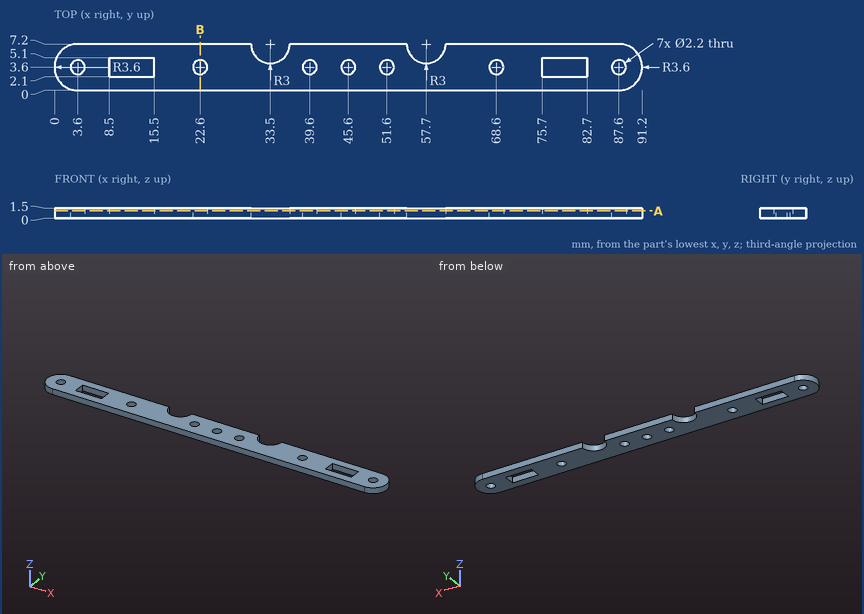
The figure shows three views and two pictorial views of one solid part (mm, origin at its lowest corner). Answer the questions. Coordinates: 2 decimals unless noted, no trailing zeros. Order: outer loops, then holes, each group sorted by start corner. A loop starts at its lowest first (then second) coordinate and runs counter-clockwise, first axis right, second up. Notation, with made-up numbers: (56, 66) - (76, 66) arc R19 cw to (76, 83) - close; hole circle Ø1 at (49.5, -5.75). An arc over 180 degrees is marked (long way). Answer as a JSON object with one key per item and string values.
1. Find section A-A on z = 1.1. Count the separate pieces of the cut face and the enclosed holes in it, plus the area to 3 significant figures.
Output values:
{"separate pieces": "1", "enclosed holes": "9", "area": "549 mm²"}
2. Consider line 1 (Y direction, x = 45.6, z = 0.45); line 2 (X direction, y = 5, z = 1.2); line 3 (Y direction, x = 9, z = 0.3). Determine where each line is inside the solid, lowest interval first.
Output values:
{"line 1": "y = 0 to 2.5, 4.7 to 7.2", "line 2": "x = 0.28 to 8.5, 15.5 to 31.46, 35.54 to 55.66, 59.74 to 75.7, 82.7 to 90.92", "line 3": "y = 0 to 2.1, 5.1 to 7.2"}
3. Find section B-B on x = 22.6. Determine the outline of the cut face in (y, z), plus the area to 3 significant figures.
Output values:
{"outline": "(0, 0) - (2.5, 0) - (2.5, 1.5) - (0, 1.5) - close; (4.7, 0) - (7.2, 0) - (7.2, 1.5) - (4.7, 1.5) - close", "area": "7.50 mm²"}
